Input: dimensioned drawing with shaded views. Units: mm. Origin: part minimum x, y, z. Round coordinates to 2 decimals unless told otherwise and drop trailing zeros. Loops run counter-clockwise (first coordinate to the right, second up) from the corner with the lowest first, then second, coordinate; pieces in that order, holes last. Notation, with made-up numbers: (73, -6.5) - (100, -6.5) arc R30 ccw to (100, 15.5) - close; hole circle Ø5 at (38, 70). An arc over 180 degrees is marked (long way). Answer as CSV lines item,"result".
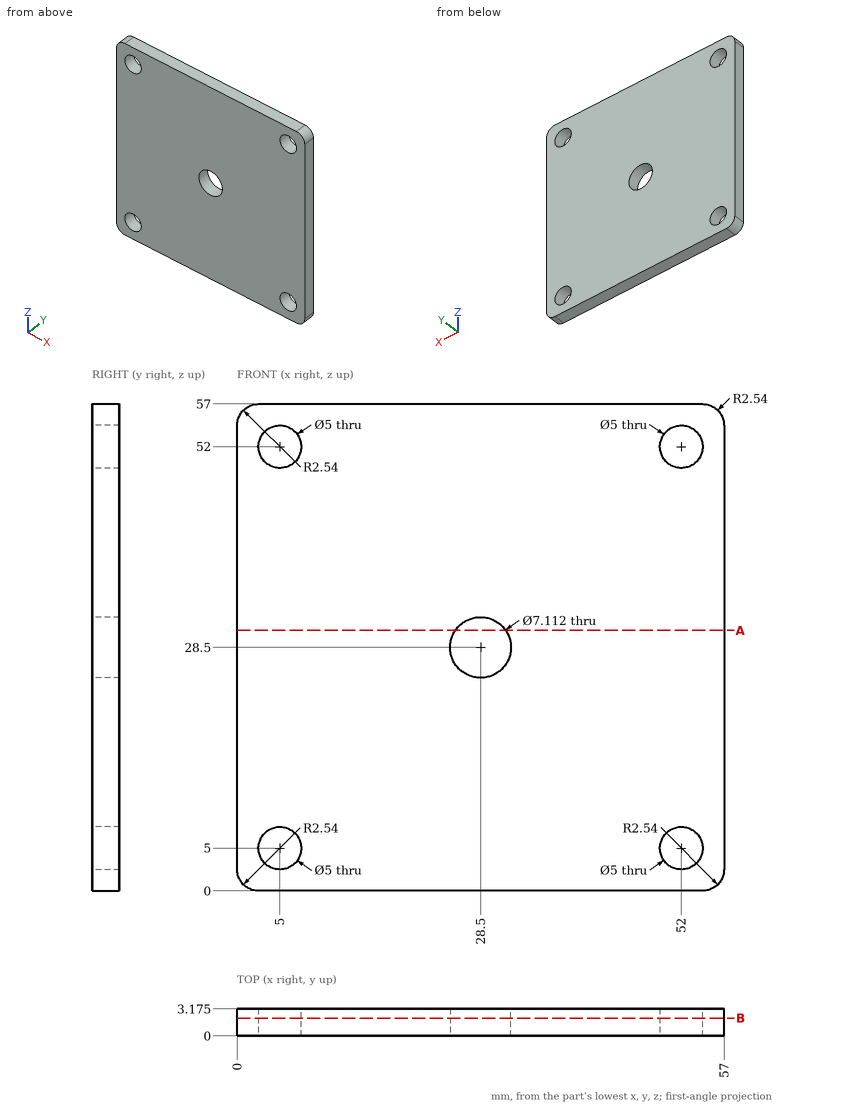
(1) Material intervals for line 1 along Z through (x, y) = (5, 0.9); line 2 along X through (y, z) = (1.5, 53); line 3 along X through (y, z) = (0.25, 31), sorted ascending.
Findings below:
line 1,"0 to 2.5, 7.5 to 49.5, 54.5 to 57"
line 2,"0 to 2.71, 7.29 to 49.71, 54.29 to 57"
line 3,"0 to 25.97, 31.03 to 57"
(2) Section A-A (z = 30.5). Output: boundary loops of the cut face in (x, y) (3 decimals).
Findings below:
outline,"(0, 0) - (25.56, 0) - (25.56, 3.175) - (0, 3.175) - close; (31.44, 0) - (57, 0) - (57, 3.175) - (31.44, 3.175) - close"
(3) Section B-B (y = 2.1). Output: boundary loops of the cut face in (x, z), and give its area (3 significant figures).
Findings below:
outline,"(0, 2.54) arc R2.54 ccw to (2.54, 0) - (54.46, 0) arc R2.54 ccw to (57, 2.54) - (57, 54.46) arc R2.54 ccw to (54.46, 57) - (2.54, 57) arc R2.54 ccw to (0, 54.46) - close; hole circle Ø5 at (5, 5); hole circle Ø5 at (5, 52); hole circle Ø7.11 at (28.5, 28.5); hole circle Ø5 at (52, 5); hole circle Ø5 at (52, 52)"
area,"3,130 mm2"
